from build123d import *

# Parameters (mm, degrees)
SKETCH1_W                                       = 80
SKETCH1_H                                       = 12.7
BASE_SHAPE_DEPTH                                = 12
CSK_FOR_M4_FLAT_HEAD_MACHINE_SCREW1_D           = 4.3
CSK_FOR_M4_FLAT_HEAD_MACHINE_SCREW1_CSINK_D     = 5
CSK_FOR_M4_FLAT_HEAD_MACHINE_SCREW1_CSINK_ANGLE = 90
CSK_FOR_M5_COUNTERSUNK_FLAT_HEAD1_D             = 5.5
CSK_FOR_M5_COUNTERSUNK_FLAT_HEAD1_CSINK_D       = 6
CSK_FOR_M5_COUNTERSUNK_FLAT_HEAD1_CSINK_ANGLE   = 90


with BuildPart() as part:
    # Sketch1 → Base Shape (new body)
    with BuildSketch(Plane.XY):
        with Locations((-40, 6.35)):
            Rectangle(SKETCH1_W, SKETCH1_H)
        with BuildLine():
            ThreePointArc((-40, 4.35), (-44, 6.35), (-40, 8.35))
            ThreePointArc((-40, 8.35), (-37.381966011, 8.586067977), (-36, 6.35))
            ThreePointArc((-36, 6.35), (-37.381966011, 4.113932023), (-40, 4.35))
        make_face(mode=Mode.SUBTRACT)
    extrude(amount=BASE_SHAPE_DEPTH)

    # CSK for M4 Flat Head Machine Screw1 (through all)
    with Locations(Plane(origin=(0, 12.7, 0), x_dir=(1, 0, 0), z_dir=(0, 1, 0))):
        with Locations((-75, -5.958952658), (-60, -5.958952658)):
            CounterSinkHole(CSK_FOR_M4_FLAT_HEAD_MACHINE_SCREW1_D / 2, CSK_FOR_M4_FLAT_HEAD_MACHINE_SCREW1_CSINK_D / 2, counter_sink_angle=CSK_FOR_M4_FLAT_HEAD_MACHINE_SCREW1_CSINK_ANGLE)

    # CSK for M5 Countersunk Flat Head1 (through all)
    with Locations(Plane(origin=(0, 0, 0), x_dir=(-1, 0, 0), z_dir=(0, -1, 0))):
        with Locations((20, -6), (5, -6)):
            CounterSinkHole(CSK_FOR_M5_COUNTERSUNK_FLAT_HEAD1_D / 2, CSK_FOR_M5_COUNTERSUNK_FLAT_HEAD1_CSINK_D / 2, counter_sink_angle=CSK_FOR_M5_COUNTERSUNK_FLAT_HEAD1_CSINK_ANGLE)


solid = part.part
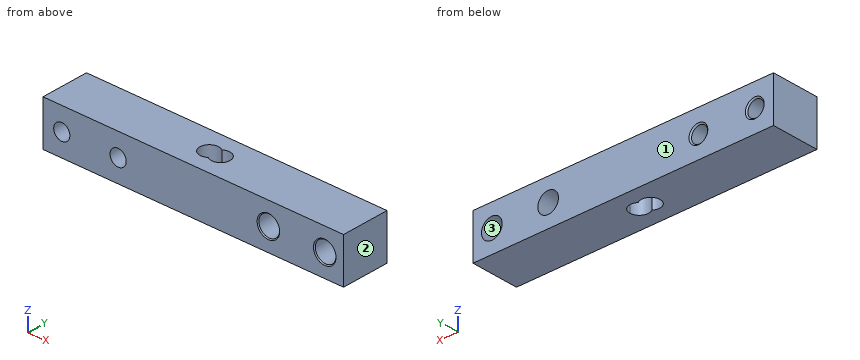
Geometry: final body of the model. Coordinates: model frame, mm. Face numbers are marked on the shaded views. Give positions to 0.01 mm unless a question says otherwise; leave off trailing zeros. Write each loop counter-clockwise with the first axis right and the second up, starting at its lowest first coordinate (ties: lowest second). Pieces come first, ordered by that corner, then holes. Notation, with made-up numbers: M -30,47 L -9,47 A20 ccw -9,79 Z; hole C 6.5,75 d7. An arc over 180 degrees is marked long. Answer in a Markdown table with one row per item. Add a question column.
(1) Section D-D on x = -60. Return loops of the section in (y, z), and give its area (3 significant figures).
(2) Ray query, line 1 (Z direction, x = -5, y = 5.75); line 2 (X direction, y = 5.75, z = 6.75); line 3 (X direction, y = 11.25, z = 7.5). Return the intervals inside material, ascending.
(3) Section A-A on x = -5. Return loops of the section in (y, z).
(4) First-contact query: pin 1 (5 mm diameter, centred on x = -17, z = 7, fed in from -Y). Flat tip, straight axial feed; report the tip coordinate or a pass-through.
(5) Section B-B on y = 7.5. Return loops of the section in (x, z), and give its area (3 significant figures).
(6) Section C-C on y = 10.75. Return loops of the section in (x, z), and give its area (3 significant figures).
(7) Mould query, pull axis X, two halves, no side actions, for the marked faces 1, 2 and 3. Classes: +X half, -X half, draft (parallel to the pull), parting line (faces both ways), or undercut.
Result set:
| question | item | result |
|---|---|---|
| 1 | outline | M 0,0 L 12.7,0 L 12.7,3.46 L 12.35,3.81 L 0,3.81 Z; M 0,8.11 L 12.35,8.11 L 12.7,8.46 L 12.7,12 L 0,12 Z |
| 1 | area | 97.7 mm^2 |
| 2 | line 1 | z = 0 to 3.25, 8.75 to 12 |
| 2 | line 2 | x = -80 to -77, -73 to -62, -58 to -43.93, -36.07 to -22.65, -17.35 to -7.65, -2.35 to 0 |
| 2 | line 3 | x = -80 to -76.5, -73.5 to -61.5, -58.5 to -22.3, -17.7 to -7.3, -2.7 to 0 |
| 3 | outline | M 0,0 L 12.7,0 L 12.7,3.25 L 0.25,3.25 L 0,3 Z; M 0,9 L 0.25,8.75 L 12.7,8.75 L 12.7,12 L 0,12 Z |
| 4 | pin 1 | stops at y = 0 |
| 5 | outline | M -80,0 L -43.72,0 L -43.72,12 L -80,12 Z; M -36.28,0 L 0,0 L 0,12 L -36.28,12 Z; hole C -75,5.96 d4.3; hole C -60,5.96 d4.3; hole C -20,6 d5.5; hole C -5,6 d5.5 |
| 5 | area | 794 mm^2 |
| 6 | outline | M -80,0 L 0,0 L 0,12 L -80,12 Z; hole C -75,5.96 d4.3; hole C -60,5.96 d4.3; hole C -20,6 d5.5; hole C -5,6 d5.5 |
| 6 | area | 883 mm^2 |
| 7 | face 1 | draft |
| 7 | face 2 | +X half |
| 7 | face 3 | undercut |
